Source: CAD feature listing. Evaluate the final solid. Frame: model axes, mm. Face numbers are marked on the shaded views. Round coordinates to 2 decimals unless told otherwise and drop trailing zeros. Loops run counter-clockwise (first coordinate to the right, second up) from the corner with the lowest first, then second, coordinate; pieces in that order, holes last. Notation, with made-up numbers: M 6,35 L 55,35 A37 cw 55,72 Z; hole C 35,-31 d2. An arc over 180 degrees is marked long. Write each question's results on one line, items separated by ' | '. Start each with the question number.
1. Ray query, line 1 (Z direction, x = 11, y = -13.5); line 2 (Z direction, x = -0.5, y = -11); line 3 (Y direction, x = 8.5, z = 1). Return the intervals inside material, ascending.
2. Section A-A on z = 0. Output: boundary loops of the cut face in (x, y).
3. Contact query for flat-ended pins moving along their axis: pin 1 Ø5 at (x, z) = (7.5, -6.5) entering from -Y; pin 2 Ø6 at (x, z) = (2.5, 4) entering from +Y; pin 3 Ø8 at (y, z) = (10, 0.5) entering from -X; pin 4 Ø3 at (x, z) = (4, -5.5) entering from +Y. Output: stop coordinate, or through.
4. Section C-C on x = 1.5. Output: boundary loops of the cut face in (y, z), and give its area (3 significant figures).
5. Section D-D on x = 11.75. Output: boundary loops of the cut face in (y, z), and give its area (3 significant figures).
6. Draft query along Y for the marked faces 1 and 2. Return one class per face: released by +Y, released by -Y, zero draft, split by the parting line, or undercut.
Solid Edge part; units mm, degrees
sketch "Sketch1" plane through (0, 0, 0) normal (0, 0, 1) x (1, 0, 0)
  arc A0 (-1.219, 16.2523) -> (-1.2597, 16.1795) centre (-1.2017, 16.1949) ccw
  line L0 (-1.2597, 16.1795) -> (-0.8903, 14.7848)
  line L1 (-0.8903, 14.7848) -> (0.0678, 15.0731)
  line L2 (0.0678, 15.0731) -> (-0.0504, 15.5193)
  arc A1 (-0.0504, 15.5193) -> (-0.0232, 15.5679) centre (-0.0117, 15.5296) cw
  line L3 (-0.0232, 15.5679) -> (13.1616, 19.536)
  line L4 (13.1616, 19.536) -> (12.9055, 20.5032)
  line L5 (12.9055, 20.5032) -> (-1.219, 16.2523)
revolve "RevolvedProtrusion1" add sketch "Sketch1" angle 360 about axis through (50, 0, 0) along (-1, 0, 0)
properties part number "320/22 X_cage"
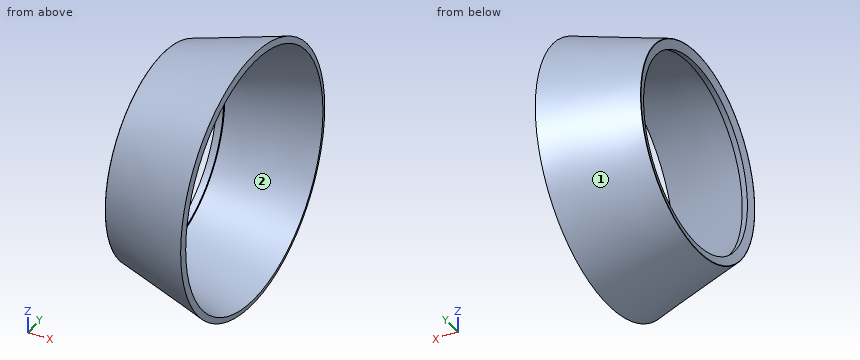
Taken from the geometry:
1) line 1: -14.66 to -13.21, 13.21 to 14.66 | line 2: -12.26 to -10.05, 10.05 to 12.26 | line 3: -19.15 to -18.11, 18.11 to 19.15
2) outline: M -1.26,-16.18 A0.06 ccw -1.22,-16.25 L 12.91,-20.5 L 13.16,-19.54 L -0.02,-15.57 A0.04 cw -0.05,-15.52 L 0.07,-15.07 L -0.89,-14.78 Z; M -1.26,16.18 L -0.89,14.78 L 0.07,15.07 L -0.05,15.52 A0.04 cw -0.02,15.57 L 13.16,19.54 L 12.91,20.5 L -1.22,16.25 A0.06 ccw Z
3) pin 1: y = -18.83 | pin 2: y = 17.98 | pin 3: through | pin 4: y = 17.59
4) outline: C 0,0 d34.14; hole C 0,0 d32.05 | area: 109 mm^2
5) outline: C 0,0 d40.31; hole C 0,0 d38.22 | area: 129 mm^2
6) face 1: split by the parting line | face 2: undercut
